For this review, take the finished solid that the model builds, in its own axes (mm). Face numbers are marked on the shaded views. A direction names the side the tool comes from. Give positions to 0.01 mm unless a question says otherwise; leave off trailing zeros. Write each loop counter-clockwise with the first axis right and the second up, starting at its lowest first coordinate (ties: lowest second). Pieces come first, ordered by that corner, then holes. Notation, with made-up numbers: (-12, 46.25) -> (40, 46.25) arc R23 ccw to (40, 62.25) -> close; hole circle Ø6 at (3, 75). An arc over 180 degrees is marked (long way). Answer as CSV lines item,"result".
```python
from build123d import *

# Parameters (mm, degrees)
SKETCH1_W                    = 530
SKETCH1_H                    = 680
BOSS_EXTRUDE1_DEPTH          = 12
BOSS_EXTRUDE2_START          = 220
SKETCH2_W                    = 510
SKETCH2_H                    = 100
BOSS_EXTRUDE2_DEPTH          = 5
BOSS_EXTRUDE3_START          = -220
SKETCH3_W                    = 510
SKETCH3_H                    = 100
BOSS_EXTRUDE3_DEPTH          = 5
SKETCH4_W                    = 50
SKETCH4_H                    = 100
SKETCH4_W_2                  = 44
SKETCH4_H_2                  = 94
EXTRUDE_THIN1_DEPTH          = 440
EXTRUDE_THIN1_2_DEPTH        = 440
SKETCH5_W                    = 530
SKETCH5_H                    = 642
BOSS_EXTRUDE4_DEPTH          = 62
SHELL1_T                     = -9
SHELL1_THICKNESS_2_FACE_W    = 624
SHELL1_THICKNESS_2_FACE_H    = 512
SHELL1_THICKNESS_2_DEPTH     = 3
SHELL1_THICKNESS_3_FACE_W    = 512
SHELL1_THICKNESS_3_FACE_H    = 50
SHELL1_THICKNESS_3_DEPTH     = 3
SHELL1_THICKNESS_4_FACE_W    = 512
SHELL1_THICKNESS_4_FACE_H    = 50
SHELL1_THICKNESS_4_DEPTH     = 3
FILLET1_R                    = 6
FILLET2_R                    = 9
FILLET3_R                    = 6
FILLET4_R                    = 9
SKETCH6_W                    = 530
SKETCH6_H                    = 6
CUT_EXTRUDE1_DEPTH           = 27.8
SKETCH7_W                    = 220
SKETCH7_H                    = 70
CUT_EXTRUDE2_DEPTH           = 748.575414256
SKETCH8_R                    = 50
CUT_EXTRUDE3_DEPTH           = 741.270896362
SKETCH9_R                    = 15
CUT_EXTRUDE4_DEPTH           = 857.023364167
M5X0_8_TAPPED_HOLE1_D        = 4.2
M5X0_8_TAPPED_HOLE1_DEPTH    = 12
LPATTERN1_COUNT              = 2
LPATTERN1_PITCH              = 600
F_7_0_7_DIAMETER_HOLE1_D     = 7
F_7_0_7_DIAMETER_HOLE1_DEPTH = 12
LPATTERN2_COUNT              = 2
LPATTERN2_PITCH              = 470
LPATTERN2_COPY_1_D           = 7
LPATTERN2_COPY_1_DEPTH       = 12
FILLET5_R                    = 30


with BuildPart() as part:
    # Sketch1 → Boss-Extrude1 (new body)
    with BuildSketch(Plane(origin=(0, 0, 0), x_dir=(1, 0, 0), z_dir=(0, 1, 0))):
        with Locations((0, 340)):
            Rectangle(SKETCH1_W, SKETCH1_H)
    extrude(amount=BOSS_EXTRUDE1_DEPTH)

    # Sketch2 → Boss-Extrude2 (add)
    with BuildSketch(Plane(origin=(0, 0, 0), x_dir=(0, 0, -1), z_dir=(1, 0, 0)).offset(BOSS_EXTRUDE2_START)):
        with Locations((340, 62)):
            Rectangle(SKETCH2_W, SKETCH2_H)
    extrude(amount=BOSS_EXTRUDE2_DEPTH)

    # Sketch3 → Boss-Extrude3 (add)
    with BuildSketch(Plane(origin=(0, 0, 0), x_dir=(0, 0, -1), z_dir=(1, 0, 0)).offset(BOSS_EXTRUDE3_START)):
        with Locations((340, 62)):
            Rectangle(SKETCH3_W, SKETCH3_H)
    extrude(amount=-BOSS_EXTRUDE3_DEPTH)


with BuildPart() as body_2:
    # Sketch4 → Extrude-Thin1 (new body)
    with BuildSketch(Plane(origin=(-220, 0, 0), x_dir=(0, 0, -1), z_dir=(1, 0, 0))):
        with Locations((160, 62)):
            Rectangle(SKETCH4_W, SKETCH4_H)
        with Locations((160, 62)):
            Rectangle(SKETCH4_W_2, SKETCH4_H_2, mode=Mode.SUBTRACT)
    extrude(amount=EXTRUDE_THIN1_DEPTH)

    # Fillet1
    fillet1_edges = [body_2.edges().sort_by_distance(p)[0] for p in [
        (0, 109, -182),
        (0, 109, -138),
        (0, 15, -182),
        (0, 15, -138),
    ]]
    fillet(fillet1_edges, radius=FILLET1_R)

    # Fillet2
    fillet2_edges = [body_2.edges().sort_by_distance(p)[0] for p in [
        (0, 112, -135),
        (0, 112, -185),
        (0, 12, -185),
        (0, 12, -135),
    ]]
    fillet(fillet2_edges, radius=FILLET2_R)


with BuildPart() as body_3:
    # Sketch4 → Extrude-Thin1 2 (new body)
    with BuildSketch(Plane(origin=(-220, 0, 0), x_dir=(0, 0, -1), z_dir=(1, 0, 0))):
        with Locations((520, 62)):
            Rectangle(SKETCH4_W, SKETCH4_H)
        with Locations((520, 62)):
            Rectangle(SKETCH4_W_2, SKETCH4_H_2, mode=Mode.SUBTRACT)
    extrude(amount=EXTRUDE_THIN1_2_DEPTH)

    # Fillet3
    fillet3_edges = [body_3.edges().sort_by_distance(p)[0] for p in [
        (0, 109, -542),
        (0, 109, -498),
        (0, 15, -542),
        (0, 15, -498),
    ]]
    fillet(fillet3_edges, radius=FILLET3_R)

    # Fillet4
    fillet4_edges = [body_3.edges().sort_by_distance(p)[0] for p in [
        (0, 112, -495),
        (0, 112, -545),
        (0, 12, -545),
        (0, 12, -495),
    ]]
    fillet(fillet4_edges, radius=FILLET4_R)


with BuildPart() as body_4:
    # Sketch5 → Boss-Extrude4 (new body)
    with BuildSketch(Plane(origin=(0, 112, 0), x_dir=(1, 0, 0), z_dir=(0, 1, 0))):
        with Locations((0, 340)):
            Rectangle(SKETCH5_W, SKETCH5_H)
    extrude(amount=BOSS_EXTRUDE4_DEPTH)

    # Shell1
    shell1_openings = [body_4.faces().sort_by_distance(p)[0] for p in [
        (0, 174, -340),
    ]]
    offset(amount=SHELL1_T, openings=shell1_openings, kind=Kind.INTERSECTION)

    # Shell1 thickness 2 face (on inner face of the shell) → Shell1 thickness 2 (add)
    with BuildSketch(Plane(origin=(0, 121, -340), x_dir=(0, 0, -1), z_dir=(0, -1, 0))):
        Rectangle(SHELL1_THICKNESS_2_FACE_W, SHELL1_THICKNESS_2_FACE_H)
    extrude(amount=-SHELL1_THICKNESS_2_DEPTH)

    # Shell1 thickness 3 face (on inner face of the shell) → Shell1 thickness 3 (cut)
    with BuildSketch(Plane(origin=(0, 149, -28), x_dir=(1, 0, 0), z_dir=(0, 0, 1))):
        Rectangle(SHELL1_THICKNESS_3_FACE_W, SHELL1_THICKNESS_3_FACE_H)
    extrude(amount=SHELL1_THICKNESS_3_DEPTH, mode=Mode.SUBTRACT)

    # Shell1 thickness 4 face (on inner face of the shell) → Shell1 thickness 4 (cut)
    with BuildSketch(Plane(origin=(0, 149, -652), x_dir=(-1, 0, 0), z_dir=(0, 0, -1))):
        Rectangle(SHELL1_THICKNESS_4_FACE_W, SHELL1_THICKNESS_4_FACE_H)
    extrude(amount=SHELL1_THICKNESS_4_DEPTH, mode=Mode.SUBTRACT)

    # Combine1: union body 2, body 3, part
    add(body_2.part)
    add(body_3.part)
    add(part.part)

    # Sketch6 → Cut-Extrude1 (cut)
    with BuildSketch(Plane(origin=(0, 174, 0), x_dir=(1, 0, 0), z_dir=(0, 1, 0))):
        with Locations((0, 22)):
            Rectangle(SKETCH6_W, SKETCH6_H)
        with Locations((0, 658)):
            Rectangle(SKETCH6_W, SKETCH6_H)
    extrude(amount=-CUT_EXTRUDE1_DEPTH, mode=Mode.SUBTRACT)

    # Sketch7 → Cut-Extrude2 (cut, through all)
    with BuildSketch(Plane(origin=(0, 12, 0), x_dir=(1, 0, 0), z_dir=(0, 1, 0))):
        with Locations((-155, 35)):
            Rectangle(SKETCH7_W, SKETCH7_H)
        with Locations((155, 35)):
            Rectangle(SKETCH7_W, SKETCH7_H)
        with Locations((155, 645)):
            Rectangle(SKETCH7_W, SKETCH7_H)
        with Locations((-155, 645)):
            Rectangle(SKETCH7_W, SKETCH7_H)
    extrude(amount=-CUT_EXTRUDE2_DEPTH, mode=Mode.SUBTRACT)

    # Sketch8 → Cut-Extrude3 (cut, through all)
    with BuildSketch(Plane(origin=(0, 124, 0), x_dir=(1, 0, 0), z_dir=(0, 1, 0))):
        with Locations(Location((0, 340, 0), (0, 0, 270))):
            Circle(SKETCH8_R)
    extrude(amount=-CUT_EXTRUDE3_DEPTH, mode=Mode.SUBTRACT)

    # Sketch9 → Cut-Extrude4 (cut, through all)
    with BuildSketch(Plane(origin=(225, 0, 0), x_dir=(0, 0, -1), z_dir=(1, 0, 0))):
        with Locations((165, 62)):
            Circle(SKETCH9_R)
        with Locations((515, 62)):
            Circle(SKETCH9_R)
    extrude(amount=-CUT_EXTRUDE4_DEPTH, mode=Mode.SUBTRACT)

    # M5x0.8 Tapped Hole1
    with Locations(Plane(origin=(0, 12, 0), x_dir=(-1, 0, 0), z_dir=(0, 1, 0))):
        with Locations((-24, -12.5), (24, -12.5), (-24, -67.5), (24, -67.5)):
            m5x0_8_tapped_hole1 = Hole(M5X0_8_TAPPED_HOLE1_D / 2, depth=M5X0_8_TAPPED_HOLE1_DEPTH)

    # LPattern1: M5x0.8 Tapped Hole1 ×2
    with Locations(*[(0, 0, -i * LPATTERN1_PITCH) for i in range(1, LPATTERN1_COUNT)]):
        add(m5x0_8_tapped_hole1, mode=Mode.SUBTRACT)

    # Ø7.0 (7) Diameter Hole1
    with Locations(Plane(origin=(0, 12, 0), x_dir=(-1, 0, 0), z_dir=(0, 1, 0))):
        with Locations((-200, -122.5), (-200, -87.5), (-250, -122.5), (-250, -87.5)):
            f_7_0_7_diameter_hole1 = Hole(F_7_0_7_DIAMETER_HOLE1_D / 2, depth=F_7_0_7_DIAMETER_HOLE1_DEPTH)

    # Mirror1: Ø7.0 (7) Diameter Hole1 across plane
    add(f_7_0_7_diameter_hole1.mirror(Plane(origin=(0, 0, 0), x_dir=(0, 0, 1), z_dir=(1, 0, 0))), mode=Mode.SUBTRACT)

    # LPattern2: Ø7.0 (7) Diameter Hole1 ×2
    with Locations(*[(0, 0, -i * LPATTERN2_PITCH) for i in range(1, LPATTERN2_COUNT)]):
        add(f_7_0_7_diameter_hole1, mode=Mode.SUBTRACT)

    # LPattern2 copy 1
    with Locations(Plane(origin=(0, 12, -470), x_dir=(1, 0, 0), z_dir=(0, 1, 0))):
        with Locations((-200, 122.5), (-200, 87.5), (-250, 122.5), (-250, 87.5)):
            Hole(LPATTERN2_COPY_1_D / 2, depth=LPATTERN2_COPY_1_DEPTH)

    # Fillet5
    fillet5_edges = [body_4.edges().sort_by_distance(p)[0] for p in [
        (-45, 6, -70),
        (45, 6, -70),
        (45, 6, -610),
        (-45, 6, -610),
    ]]
    fillet(fillet5_edges, radius=FILLET5_R)


solid = body_4.part
```
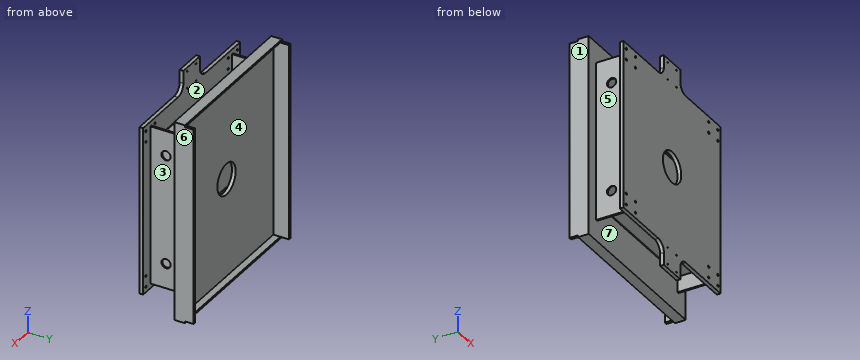
Q1. Add section B-B (z = -165). Write out the cut boundary in (x, y), plus the area to 3 significant figures.
Answer block:
outline,"(-265, 0) -> (265, 0) -> (265, 12) -> (225, 12) -> (225, 47) -> (220, 47) -> (220, 15) -> (-220, 15) -> (-220, 47) -> (-225, 47) -> (-225, 12) -> (-265, 12) -> close; (-265, 112) -> (-225, 112) -> (-225, 77) -> (-220, 77) -> (-220, 109) -> (220, 109) -> (220, 77) -> (225, 77) -> (225, 112) -> (265, 112) -> (265, 174) -> (256, 174) -> (256, 124) -> (-256, 124) -> (-256, 174) -> (-265, 174) -> close"
area,"17,000 mm2"
Q2. Add section C-C (x = -10.5). State how many separate pieces and enclosed holes the cut face has, plus the area to 3 significant figures.
Answer block:
separate pieces,"2"
enclosed holes,"2"
area,"15,400 mm2"
Q3. To check wall thickness, follow probe 1 along X at (y, z) = (7, -557.5); probe 2 along Z at (x, y) = (160.5, 29); probe 3 along Y at (x, z) = (-109, -367.5). State the ranges of each line that lie inside material, in increasing order. Write a range as [from, to].
Answer block:
probe 1,"x = [-265, -253.5], [-246.5, -203.5], [-196.5, 196.5], [203.5, 246.5], [253.5, 265]"
probe 2,"z = [-545, -542], [-498, -495], [-185, -182], [-138, -135]"
probe 3,"y = [0, 12], [112, 124]"
Q4. Draft analysis for pull direction X (two halves, no side actions). For the marked faces 1, 2 and 3, state which applies: released by +X, released by -X, zero draft, split by the parting line, or undercut.
Answer block:
face 1,"released by -X"
face 2,"undercut"
face 3,"released by +X"
Q5. For the marked faces 4, 5, 6 and 7, list the 3-axis set-ups (+Z, -Z, +X, -X, +Y, -Y) from which the entire face can be reached by the end or side of a thin tool; tool diameter is ignored.
Answer block:
face 4,"+Y"
face 5,"+Z, -Z, -X"
face 6,"+Z, -Z, +X, +Y, -Y"
face 7,"none"
Q6. Add section A-A (x = -233). Write out the cut boundary in (y, z).
Answer block:
outline,"(0, -610) -> (12, -610) -> (12, -70) -> (0, -70) -> close; (112, -661) -> (146.2, -661) -> (146.2, -655) -> (124, -655) -> (124, -25) -> (146.2, -25) -> (146.2, -19) -> (112, -19) -> close"
Q7. Clearance check with flat-ended pins moving along their axes: pin 1 (2.5 mm diameter, centred on x = -24, z = -612.5, fed in from -Y); pin 2 (6 mm diameter, centred on y = 64, z = -577.5, fed in from +X); pin 3 (4.5 mm diameter, centred on x = -258.5, y = 166, fed in from -Z). State where each tip first meets the part, or that it passes through.
Answer block:
pin 1,"stops at y = 112"
pin 2,"stops at x = 225"
pin 3,"stops at z = -655"
